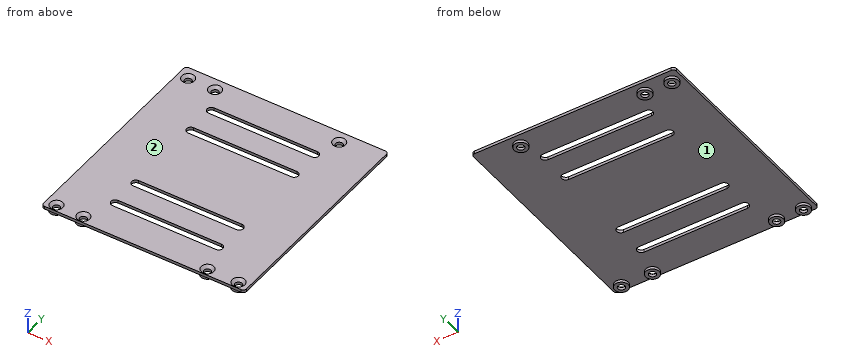
from build123d import *

# Parameters (mm, degrees)
PAD009_DEPTH     = 1.4
SKETCH015_R      = 3.25
PAD010_DEPTH     = 2.7
HOLE_D           = 3.4
HOLE_DEPTH       = 25
HOLE_CSINK_D     = 6.1
HOLE_CSINK_ANGLE = 90
POCKET003_DEPTH  = 1.4


with BuildPart() as part:
    # Sketch014 → Pad009 (new body)
    with BuildSketch(Plane.XY):
        with BuildLine():
            Line((-49, 51), (-49, -51))
            ThreePointArc((-49, -51), (-48.56066, -52.06066), (-47.5, -52.5))
            Line((-47.5, -52.5), (47.5, -52.5))
            ThreePointArc((47.5, -52.5), (48.56066, -52.06066), (49, -51))
            Line((49, -51), (49, 51))
            ThreePointArc((49, 51), (48.56066, 52.06066), (47.5, 52.5))
            Line((47.5, 52.5), (-47.5, 52.5))
            ThreePointArc((-47.5, 52.5), (-48.56066, 52.06066), (-49, 51))
        make_face()
    extrude(amount=-PAD009_DEPTH)

    # Sketch015 → Pad010 (join)
    with BuildSketch(Plane.XY):
        with Locations((-44, 46.766667)):
            Circle(SKETCH015_R)
        with Locations((-31, 46.766667)):
            Circle(SKETCH015_R)
        with Locations((29, 46.766667)):
            Circle(SKETCH015_R)
        with Locations((-44, -49.166667)):
            Circle(SKETCH015_R)
        with Locations((-31, -49.166667)):
            Circle(SKETCH015_R)
        with Locations((29, -49.166667)):
            Circle(SKETCH015_R)
        with Locations((44, -49.166667)):
            Circle(SKETCH015_R)
    extrude(amount=-PAD010_DEPTH)

    # Hole
    with Locations(Plane.XY):
        with Locations((-44, 46.766667), (-31, 46.766667), (29, 46.766667), (-44, -49.166667), (-31, -49.166667), (29, -49.166667), (44, -49.166667)):
            CounterSinkHole(HOLE_D / 2, HOLE_CSINK_D / 2, depth=HOLE_DEPTH, counter_sink_angle=HOLE_CSINK_ANGLE)

    # Sketch016 (on Face4 of Hole) → Pocket003 (cut)
    with BuildSketch(Plane.XY):
        with BuildLine():
            ThreePointArc((-25, 37), (-27, 35), (-25, 33))
            Line((-25, 33), (25, 33))
            ThreePointArc((25, 33), (27, 35), (25, 37))
            Line((-25, 37), (25, 37))
        make_face()
        with BuildLine():
            ThreePointArc((-25, -33), (-27, -35), (-25, -37))
            Line((-25, -37), (25, -37))
            ThreePointArc((25, -37), (27, -35), (25, -33))
            Line((-25, -33), (25, -33))
        make_face()
        with BuildLine():
            ThreePointArc((-25, 22), (-27, 20), (-25, 18))
            Line((-25, 18), (25, 18))
            ThreePointArc((25, 18), (27, 20), (25, 22))
            Line((-25, 22), (25, 22))
        make_face()
        with BuildLine():
            ThreePointArc((-25, -18), (-27, -20), (-25, -22))
            Line((-25, -22), (25, -22))
            ThreePointArc((25, -22), (27, -20), (25, -18))
            Line((-25, -18), (25, -18))
        make_face()
    extrude(amount=-POCKET003_DEPTH, mode=Mode.SUBTRACT)


with BuildPart() as part_1:
    # Body003 placement: moved
    add(part.part.moved(Location((0, 0, 63.5))))


solid = part_1.part
CAD build for the part. Positions are in the model's coordinates, mm. Face numbers are marked on the shaded views. Round coordinates to 2 decimals unless told otherwise and drop trailing zeros. Write each loop counter-clockwise with the first axis right and the second up, starting at its lowest first coordinate (ties: lowest second). Pieces come first, ordered by that corner, then holes.
(1) Slice it at A-A, the plane y = 20. Write the cut outline in (x, z).
(2) Mould opens along X. For the marked faces 1 and 2 say: pulls with the +X half, pulls with the -X half, needs draft (parallel to the pull), parting line crosses it, or undercut.
(3) Slice it at D-D, the plane x = -31. Write the cut outline in (y, z).
(4) Slice it at C-C, the plane x = 44. Write the cut outline in (y, z), and give its area (3 significant figures).
(5) Slice it at B-B, the plane x = -9.5. Write the cut outline in (y, z), and give its area (3 significant figures).
(6) Probe line 1 along Y through (x, z) = (-44, 61.75); line 2 along Y through (x, z) = (-7.5, 63.35); line 3 along Y through (x, z) = (44, 61.5). List the from-to ranges inside material, lowest first.
(7) Drop flat-ended pins along their axis: P1, Ø1, axis at y = -12.5, z = 61, coming from the +X side; P2, Ø12, axis at x = -8, y = 27, coming from the -Z side; P3, Ø4, axis at x = -31, y = 46.77, coming from the +Z side; P4, Ø4.5, axis at x = 44, y = -49.17, coming from the +Z side. Give the stop position or say it passes through.
From the geometry:
1. outline: (-49, 62.1) - (-27, 62.1) - (-27, 63.5) - (-49, 63.5) - close; (27, 62.1) - (49, 62.1) - (49, 63.5) - (27, 63.5) - close
2. face 1: undercut
2. face 2: needs draft
3. outline: (-52.5, 62.1) - (-52.42, 62.1) - (-52.42, 60.8) - (-50.87, 60.8) - (-50.87, 62.15) - (-52.22, 63.5) - (-52.5, 63.5) - close; (-47.47, 60.8) - (-45.92, 60.8) - (-45.92, 62.1) - (43.52, 62.1) - (43.52, 60.8) - (45.07, 60.8) - (45.07, 62.15) - (43.72, 63.5) - (-46.12, 63.5) - (-47.47, 62.15) - close; (48.47, 60.8) - (50.02, 60.8) - (50.02, 62.1) - (52.5, 62.1) - (52.5, 63.5) - (49.82, 63.5) - (48.47, 62.15) - close
4. outline: (-52.5, 62.1) - (-52.42, 62.1) - (-52.42, 60.8) - (-50.87, 60.8) - (-50.87, 62.15) - (-52.22, 63.5) - (-52.5, 63.5) - close; (-47.47, 60.8) - (-45.92, 60.8) - (-45.92, 62.1) - (52.5, 62.1) - (52.5, 63.5) - (-46.12, 63.5) - (-47.47, 62.15) - close
4. area: 144 mm2
5. outline: (-52.5, 62.1) - (-37, 62.1) - (-37, 63.5) - (-52.5, 63.5) - close; (-33, 62.1) - (-22, 62.1) - (-22, 63.5) - (-33, 63.5) - close; (-18, 62.1) - (18, 62.1) - (18, 63.5) - (-18, 63.5) - close; (22, 62.1) - (33, 62.1) - (33, 63.5) - (22, 63.5) - close; (37, 62.1) - (52.5, 62.1) - (52.5, 63.5) - (37, 63.5) - close
5. area: 125 mm2
6. line 1: y = -52.42 to -50.87, -47.47 to -45.92, 43.52 to 45.07, 48.47 to 50.02
6. line 2: y = -52.5 to -37, -33 to -22, -18 to 18, 22 to 33, 37 to 52.5
6. line 3: y = -52.42 to -50.87, -47.47 to -45.92
7. P1: passes through
7. P2: stops at z = 62.1
7. P3: stops at z = 62.45
7. P4: stops at z = 62.7
